Here's how the part is built. I have some questions about the finished solid (model axes, mm). A direction names the side the tool comes from. Give positions to 0.01 mm unless a question says otherwise; leave off trailing zeros. Write each loop counter-clockwise with the first axis right and the second up, starting at its lowest first coordinate (ties: lowest second). Pieces come first, ordered by that corner, then holes. Notation, with made-up numbers: (-14, 63.5) -> (44, 63.5) arc R29 cw to (44, 85.5) -> close; hole circle Ø6 at (82.25, 58). An arc over 180 degrees is marked (long way). Use one line per item in the form item = value.
```python
from build123d import *

# Parameters (mm, degrees)
SKETCH_1_R          = 25.5
EXTRUDE_1_DEPTH     = 3.5
SKETCH_2_R          = 19
SKETCH_2_R_2        = 18.5
CUT_EXTRUDE_1_DEPTH = 2
SKETCH_3_R          = 22.1
SKETCH_3_R_2        = 21.6
CUT_EXTRUDE_2_DEPTH = 2
FILLET_1_R          = 0.4
SKETCH_4_R          = 14.809002025
CUT_EXTRUDE_3_DEPTH = 10


with BuildPart() as part:
    # 草图1 → 凸台-拉伸1 (new body)
    with BuildSketch(Plane(origin=(0, 0, 0), x_dir=(1, 0, 0), z_dir=(0, 1, 0))):
        Circle(SKETCH_1_R)
    extrude(amount=EXTRUDE_1_DEPTH)

    # 草图2 → 切除-拉伸1 (cut)
    with BuildSketch(Plane(origin=(0, 3.5, 0), x_dir=(1, 0, 0), z_dir=(0, 1, 0))):
        Circle(SKETCH_2_R)
        Circle(SKETCH_2_R_2, mode=Mode.SUBTRACT)
    extrude(amount=-CUT_EXTRUDE_1_DEPTH, mode=Mode.SUBTRACT)

    # 草图3 → 切除-拉伸2 (cut)
    with BuildSketch(Plane(origin=(0, 3.5, 0), x_dir=(1, 0, 0), z_dir=(0, 1, 0))):
        Circle(SKETCH_3_R)
        Circle(SKETCH_3_R_2, mode=Mode.SUBTRACT)
    extrude(amount=-CUT_EXTRUDE_2_DEPTH, mode=Mode.SUBTRACT)

    # 圆角1
    fillet_1_edges = [part.edges().sort_by_distance(p)[0] for p in [
        (-22.1, 3.5, 0),
        (-21.6, 3.5, 0),
        (-19, 3.5, 0),
        (-18.5, 3.5, 0),
    ]]
    fillet(fillet_1_edges, radius=FILLET_1_R)

    # 草图4 → 切除-拉伸3 (cut)
    with BuildSketch(Plane.XZ):
        Circle(SKETCH_4_R)
    extrude(amount=-CUT_EXTRUDE_3_DEPTH, mode=Mode.SUBTRACT)


solid = part.part
```
Q1. I want a section at C-C, the plane y = 0.8. Write out the boundary of the cut face in (x, z), and give its area (3 significant figures).
Result set:
outline = circle Ø51 at (0, 0); hole circle Ø29.62 at (0, 0)
area = 1,350 mm2
Q2. Which directions (+Z, -Z, +X, -X, +Y, -Y) give clear straight access to the entire face, cutting with the end or side of a thin tool? Please do faces 1 (the face through (19.5, 1.5, 9.7)), 2 (the face through (-1.928, 1.726, 14.683)).
Result set:
face_1 = +Y
face_2 = +Y, -Y
Q3. Will these pins go through, and if not, where does the flat tip stop? pin 1 Ø1.5 at (x, y) = (12, 0.5) entering from +Z; pin 2 Ø2 at (x, y) = (-17.5, 0.5) entering from -Z.
Result set:
pin_1 = 22.88
pin_2 = -19.44
Q4. If we mould it in two halves opening along Z, with no side actions, what happens to faces 3 (the face through (-5.5, 1.7, 24.9)), 4 (the face through (-15, 3.5, 0)), 5 (the face through (-4.682, 2.311, 21.086))? For each: +Z half, -Z half, draft (parallel to the pull), parting line (faces both ways), or undercut.
Result set:
face_3 = parting line
face_4 = draft
face_5 = undercut
Q5. If I drill on line 1 along Z through (x, y) = (0, 1.85); line 2 along Z through (x, y) = (0, 1.05); line 3 along Z through (x, y) = (-4, 2.35) (3 decimals), over which ranges is the centre line in solid material (lowest first)? Write a range as from..to.
Result set:
line_1 = -25.5..-22.1, -21.6..-19, -18.5..-14.81, 14.81..18.5, 19..21.6, 22.1..25.5
line_2 = -25.5..-14.81, 14.81..25.5
line_3 = -25.184..-21.735, -21.226..-18.574, -18.062..-14.259, 14.259..18.062, 18.574..21.226, 21.735..25.184
